Check sheet for the modelled part. Datum: model origin and axes. Units: mm. Give positions to 0.01 mm unless a question says otherwise; leave off trailing zeros. Order: outer loops, then holes, each group sorted by start corner. A loop starts at its lowest first (then second) coordinate and runs counter-clockwise, first axis right, second up.
from build123d import *

# Parameters (mm, degrees)
BOSS_EXTRUDE1_DEPTH = 1.5875


with BuildPart() as part:
    # Sketch1 → Boss-Extrude1 (new body)
    with BuildSketch(Plane(origin=(0, 0, 0), x_dir=(0, 0, -1), z_dir=(1, 0, 0))):
        with BuildLine():
            ThreePointArc((200, 0), (141.421356237, 141.421356237), (0, 200))
            Line((0, 200), (0, 75))
            ThreePointArc((0, 75), (53.033008589, 53.033008589), (75, 0))
            ThreePointArc((75, 0), (53.033008589, -53.033008589), (0, -75))
            Line((0, -75), (0, -200))
            ThreePointArc((0, -200), (141.421356237, -141.421356237), (200, 0))
        make_face()
    extrude(amount=BOSS_EXTRUDE1_DEPTH)


solid = part.part
1) Section check B-B, the plane x = 0.25. Record the cut outline in (y, z).
Recorded:
outline: (-200, 0) arc R200 ccw to (200, 0) - (75, 0) arc R75 cw to (-75, 0) - close
2) Material ranges on L1, parallel to Y at x = 0.45, z = -34.5; L2, parallel to Y at x = 0.6, z = -61.5; L3, parallel to Z at x = 1.15, y = -151.5, recorded low to high.
Recorded:
L1: y = -197 to -66.59, 66.59 to 197
L2: y = -190.31 to -42.93, 42.93 to 190.31
L3: z = -130.57 to 0
3) Depth check by flat-ended pin: pin 1 Ø8 at (y, z) = (63, -55) entering from -X. Enter the tip coordinate at first touch or a pass-through.
Recorded:
pin 1: stops at x = 0
4) Section check D-D, the plane y = -173. Record the cut outline in (x, z), then the cut area to 3 significant figures.
Recorded:
outline: (0, -100.35) - (1.59, -100.35) - (1.59, 0) - (0, 0) - close
area: 159 mm2
5) Section check A-A, the plane z = -60.5. Record the cut outline in (x, y), then the cut area to 3 significant figures.
Recorded:
outline: (0, -190.63) - (1.59, -190.63) - (1.59, -44.33) - (0, -44.33) - close; (0, 44.33) - (1.59, 44.33) - (1.59, 190.63) - (0, 190.63) - close
area: 465 mm2
6) Section check C-C, the plane z = -26. Record the cut outline in (x, y).
Recorded:
outline: (0, -198.3) - (1.59, -198.3) - (1.59, -70.35) - (0, -70.35) - close; (0, 70.35) - (1.59, 70.35) - (1.59, 198.3) - (0, 198.3) - close
7) Draft check along Y on faces 1 (the face through (1.588, 3, -99)), 2 (the face through (0.78, 1.65, -74.98)). Enter one of: +Y half, -Y half, draft (parallel to the pull), parting line (faces both ways), or undercut.
Recorded:
face 1: draft
face 2: undercut
